Here's how the part is built. I have some questions about the finished solid (model axes, mm). A direction names the side the tool comes from. Coordinates: 2 decimals unless noted, no trailing zeros. Order: outer loops, then holes, each group sorted by start corner. A loop starts at its lowest first (then second) coordinate and runs counter-clockwise, first axis right, second up. Notation, with made-up numbers: (-24.5, -7.5) - (23.5, -7.5) arc R24 ccw to (23.5, 24.5) - close; hole circle Ø8 at (86, 7). An arc over 180 degrees is marked (long way). Answer in a Markdown table with one row per item. Add a question column.
Item 1: I want a section at D-D (z = -15.5). Please give me the cut outline in (x, y).
Item 2: If I drill on line 1 along Z through (x, y) = (-0.9, 0); line 2 along X through (y, z) = (-17, 12); line 3 along Z through (x, y) = (0.35, -5), over which ranges is the centre line in solid material (lowest first)? Write a range as from..to.
Item 3: Will this pin go through, and if not, where does the flat tip stop? pin 1 Ø14.5 at (y, z) = (7, 0) entering from -X.
Item 4: I want a section at C-C (y = 18.5). Please give me the cut outline in (x, z).
Item 5: On a 3-axis mill with a long thin cutter (end or side, diameter ignored), from which of +Z, -Z, +X, -X, +Y, -Y can I reach the whole of each face in a straight line? I mean faces 5 (the flat face through (-0.75, 18.6, -9.2)), 6 (the flat face through (1, -5, 14)), 7 (the flat face through (0.75, 18.6, -9.2)). Say none if no direction works.
Item 6: Thinking about a two-plate mould opening in Y: for faces 1 (the cylindrical face through (-0.01, 20.03, -6.31)), 2 (the flat face through (-0.75, -11, 7)), 3 (the flat face through (-1, -5, 14)), 4 (the cylindrical face through (0.01, 11.923, 3.755)), which applies, +Y half, -Y half, draft (parallel to the pull), parting line (faces both ways), or undercut?
Item 7: I want a section at A-A (y = 0). Please give me the cut outline in (x, z), plus the area to 3 significant figures.
Autodesk Inventor part; units mm, degrees
ref_plane "core_to_washer_XY" through (0, 0, 0) normal (1, 0, 0) x (0, 0, -1)
ref_plane "core_to_washer_YZ" through (0, 0, 0) normal (0, 0, -1) x (0, 1, 0)
ref_plane "core_to_washer_ZX" through (0, 0, 0) normal (0, 1, 0) x (1, 0, 0)
sketch "Sketch_1" plane through (0, 0, 0) normal (0, 0, 1) x (1, 0, 0)
  line L0 (50, 0) -> (-50, 0)
  line L1 (-1, 20.5) -> (-1, 14.5)
  line L2 (-1, 14.5) -> (-0.75, 14.5)
  line L3 (-0.75, 14.5) -> (-0.75, 12.5)
  line L4 (-0.75, 12.5) -> (0.75, 12.5)
  line L5 (0.75, 12.5) -> (0.75, 14.5)
  line L6 (0.75, 14.5) -> (1, 14.5)
  line L7 (1, 14.5) -> (1, 20.5)
  line L8 (1, 20.5) -> (0.75, 20.5)
  line L9 (0.75, 20.5) -> (0.75, 21)
  line L10 (0.75, 21) -> (-0.75, 21)
  line L11 (-0.75, 21) -> (-0.75, 20.5)
  line L12 (-0.75, 20.5) -> (-1, 20.5)
revolve "Revolution1" add sketch "Sketch_1" angle 360 about axis through (50, 0, 0) along (1, 0, 0)
ref_plane "core_to_washer_XY" through (0, 0, 0) normal (1, 0, 0) x (0, 0, -1)
ref_plane "core_to_washer_YZ" through (0, 0, 0) normal (0, 0, -1) x (0, 1, 0)
ref_plane "core_to_washer_ZX" through (0, 0, 0) normal (0, 1, 0) x (1, 0, 0)
ref_plane "core_to_washer1_XY" through (0, 0, 0) normal (-1, 0, 0) x (0, 0, -1)
ref_plane "core_to_washer1_YZ" through (0, 0, 0) normal (0, 0, -1) x (0, -1, 0)
ref_plane "core_to_washer1_ZX" through (0, 0, 0) normal (0, -1, 0) x (-1, 0, 0)
properties part number "core_BA2542"
Values follow:
| question | item | result |
|---|---|---|
| 1 | outline | (-1, -13.42) - (-0.75, -13.42) - (-0.75, -14.17) - (0.75, -14.17) - (0.75, -13.42) - (1, -13.42) - (1, 13.42) - (0.75, 13.42) - (0.75, 14.17) - (-0.75, 14.17) - (-0.75, 13.42) - (-1, 13.42) - close |
| 2 | line 1 | z = -20.5..-14.5, 14.5..20.5 |
| 2 | line 2 | x = -0.75..0.75 |
| 2 | line 3 | z = -20.4..-11.46, 11.46..20.4 |
| 3 | pin 1 | stops at x = -0.75 |
| 4 | outline | (-1, -8.83) - (-0.75, -8.83) - (-0.75, -9.94) - (0.75, -9.94) - (0.75, -8.83) - (1, -8.83) - (1, 8.83) - (0.75, 8.83) - (0.75, 9.94) - (-0.75, 9.94) - (-0.75, 8.83) - (-1, 8.83) - close |
| 5 | face 5 | -X |
| 5 | face 6 | +Z, -Z, +X, +Y, -Y |
| 5 | face 7 | +X |
| 6 | face 1 | parting line |
| 6 | face 2 | undercut |
| 6 | face 3 | draft |
| 6 | face 4 | undercut |
| 7 | outline | (-1, -20.5) - (-0.75, -20.5) - (-0.75, -21) - (0.75, -21) - (0.75, -20.5) - (1, -20.5) - (1, -14.5) - (0.75, -14.5) - (0.75, -12.5) - (-0.75, -12.5) - (-0.75, -14.5) - (-1, -14.5) - close; (-1, 14.5) - (-0.75, 14.5) - (-0.75, 12.5) - (0.75, 12.5) - (0.75, 14.5) - (1, 14.5) - (1, 20.5) - (0.75, 20.5) - (0.75, 21) - (-0.75, 21) - (-0.75, 20.5) - (-1, 20.5) - close |
| 7 | area | 31.5 mm^2 |
